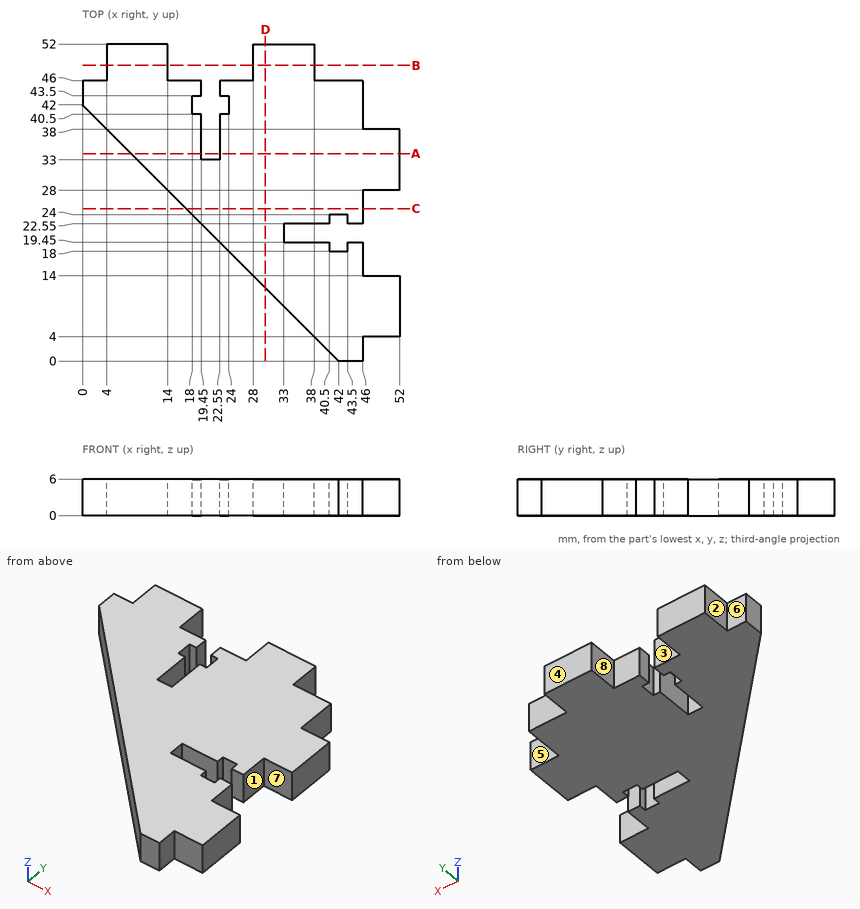
The drawing under review shows one solid part. Ordinate dimensions are in mm from its lowest x, y, z. A direction names the side the tool comes from. Give positions to 0.01 mm unless a question says otherwise; leave off trailing zeros. Write each loop counter-clockwise with the first axis right and the second up, starting at its lowest first coordinate (ties: lowest second). Pieces come first, ordered by that corner, then holes.
1. For P1, Ø2.5, axis at x = 17, z = 4, coming from the +Y side; P2, Ø1.8, axis at y = 48.5, z = 4, coming from the +X side; P3, Ø2, axis at y = 2.5, z = 3.5, coming from the +X side, all flat-tipped, find the tip position at first contact; note any pin that passes through.
2. Tool access review of the marked faces 5, 6, 7 and 8: name each direction out of +Z, -Z, +X, -X, +Y, -Y from which nothing blocks a thin tool from reaching the whole face with its end or side.
3. Add section C-C, the plane y = 25. Write out the cut boundary in (x, z), plus the area to 3 significant figures.
4. Add section B-B, the plane y = 48.5. Write out the cut boundary in (x, z), plus the area to 3 significant figures.
5. Draft analysis for pull direction X (two halves, no side actions). For the marked faces 1, 2, 3 and 4, state which applies: +X half, -X half, draft (parallel to the pull), parting line (faces both ways), or undercut.
6. Add section D-D, the plane x = 30. Write out the cut boundary in (y, z).
7. Wall thickness on L1, parallel to Y at x = 36, z = 3.8; L2, parallel to Y at x = 42.5, z = 1.1; L3, parallel to Y at x = 9, z = 0.5: over which ranges is each line inside the solid? List them lowest first.
8. Add section A-A, the plane y = 34. Write out the cut boundary in (x, z), plus the area to 3 significant figures.
Worked answers:
1. P1: stops at y = 46
1. P2: stops at x = 38
1. P3: stops at x = 46
2. face 5: +Z, -Z, +X, +Y
2. face 6: +Z, -Z, -X, +Y
2. face 7: +Z, -Z, +X
2. face 8: +Z, -Z, +Y
3. outline: (17, 0) - (46, 0) - (46, 6) - (17, 6) - close
3. area: 174 mm2
4. outline: (4, 0) - (14, 0) - (14, 6) - (4, 6) - close; (28, 0) - (38, 0) - (38, 6) - (28, 6) - close
4. area: 120 mm2
5. face 1: +X half
5. face 2: -X half
5. face 3: undercut
5. face 4: draft
6. outline: (12, 0) - (52, 0) - (52, 6) - (12, 6) - close
7. L1: y = 6 to 19.45, 22.55 to 52
7. L2: y = 0 to 18, 24 to 46
7. L3: y = 33 to 52
8. outline: (8, 0) - (19.45, 0) - (19.45, 6) - (8, 6) - close; (22.55, 0) - (52, 0) - (52, 6) - (22.55, 6) - close
8. area: 245 mm2
